Could you check a few things on this model? Use its own coordinates, in mm. A direction names the side the tool comes from. Round coordinates to 2 decimals unless told otherwise and drop trailing zeros. Loops run counter-clockwise (first coordinate to the right, second up) from the corner with the lowest first, then second, coordinate; pieces in that order, holes last.
from build123d import *

# Parameters (mm, degrees)
SKETCH1_W               = 571.5
SKETCH1_H               = 100.8
BOSS_EXTRUDE1_DEPTH     = 8
CUT_EXTRUDE1_DEPTH      = 581.541893406
CUT_EXTRUDE1_DEPTH_BACK = 581.541893406
SKETCH9_R               = 11
SKETCH9_R_2             = 2.65
SKETCH10_W              = 32
SKETCH10_H              = 30
CUT_EXTRUDE2_DEPTH      = 10
SKETCH11_R              = 7.5
CUT_EXTRUDE3_DEPTH      = 5
CUT_EXTRUDE4_START      = -11
SKETCH11_2_R            = 7.5
CUT_EXTRUDE4_DEPTH      = 5


with BuildPart() as part:
    # Sketch1 → Boss-Extrude1 (new, symmetric)
    with BuildSketch(Plane.XY):
        with Locations((285.75, 50.4)):
            Rectangle(SKETCH1_W, SKETCH1_H)
    extrude(amount=BOSS_EXTRUDE1_DEPTH, both=True)

    # Sketch9 → Cut-Extrude1 (cut, two sides: drawn at the far end of the back side and taken through both)
    with BuildSketch(Plane.XY.offset(8).offset(-CUT_EXTRUDE1_DEPTH_BACK)):
        with Locations((50, 50.4)):
            Circle(SKETCH9_R)
        with Locations((110, 80.8)):
            Circle(SKETCH9_R_2)
        with Locations((110, 50.8)):
            Circle(SKETCH9_R_2)
    extrude(amount=CUT_EXTRUDE1_DEPTH + CUT_EXTRUDE1_DEPTH_BACK, mode=Mode.SUBTRACT)

    # Sketch10 → Cut-Extrude2 (cut)
    with BuildSketch(Plane.XY.offset(8)):
        with Locations((50, 50.4)):
            Rectangle(SKETCH10_W, SKETCH10_H)
    extrude(amount=-CUT_EXTRUDE2_DEPTH, mode=Mode.SUBTRACT)

    # Sketch11 → Cut-Extrude3 (cut)
    with BuildSketch(Plane.XY.offset(8)):
        with Locations((110, 80.8)):
            Circle(SKETCH11_R)
        with Locations((110, 50.8)):
            Circle(SKETCH11_R)
    extrude(amount=-CUT_EXTRUDE3_DEPTH, mode=Mode.SUBTRACT)

    # Sketch11<2> → Cut-Extrude4 (cut)
    with BuildSketch(Plane.XY.offset(8).offset(CUT_EXTRUDE4_START)):
        with Locations((110, 80.8)):
            Circle(SKETCH11_2_R)
        with Locations((110, 50.8)):
            Circle(SKETCH11_2_R)
    extrude(amount=-CUT_EXTRUDE4_DEPTH, mode=Mode.SUBTRACT)


solid = part.part
Item 1: If we section it at A-A, the plane x = 50: Please give me the cut outline in (y, z), then the cut area to 3 significant figures.
Results list:
outline: (0, -8) - (39.4, -8) - (39.4, -2) - (35.4, -2) - (35.4, 8) - (0, 8) - close; (61.4, -8) - (100.8, -8) - (100.8, 8) - (65.4, 8) - (65.4, -2) - (61.4, -2) - close
area: 1,180 mm2
Item 2: For faces 5 (the flat face through (34, 50, 3)), 6 (the flat face through (113, 81, -3)), 7 (the flat face through (282, 100.8, 0)), which set-ups out of +Z, -Z, +X, -X, +Y, -Y let a thin tool reach every point of the face, with its end or its side?
Results list:
face 5: +Z
face 6: -Z
face 7: +Z, -Z, +X, -X, +Y
Item 3: We'd pull the mould along Y, two halves only. Please class faces 1 (the flat face through (282, 0, 0)), 2 (the cylindrical face through (117.154, 83.053, -5.465)), 3 (the flat face through (282, 51, 8)), 4 (the flat face through (113, 81, 3)): released by +Y, released by -Y, zero draft, split by the parting line, or undercut.
Results list:
face 1: released by -Y
face 2: undercut
face 3: zero draft
face 4: undercut
Item 4: Will these pins go through, and if not, where does the flat tip stop? pin 1 (9 mm diameter, centred on x = 110, y = 80.8, fed in from -Z); pin 2 (24 mm diameter, centred on x = 110, y = 50.8, fed in from +Z); pin 3 (5 mm diameter, centred on x = 110, y = 80.8, fed in from +Z); pin 4 (4.5 mm diameter, centred on x = 108, y = 80, fed in from +Z).
Results list:
pin 1: stops at z = -3
pin 2: stops at z = 8
pin 3: passes through
pin 4: stops at z = 3
Item 5: If I drill on line 1 along Y through (x, z) = (110, 6.25); line 2 along Y through (x, z) = (110, 0.9); line 3 along X through (y, z) = (81, -4.25), over which ranges is the centre line in solid material (lowest first)?
Results list:
line 1: y = 0 to 43.3, 58.3 to 73.3, 88.3 to 100.8
line 2: y = 0 to 48.15, 53.45 to 78.15, 83.45 to 100.8
line 3: x = 0 to 102.5, 117.5 to 571.5
